Source: CAD feature listing. Evaluate the final solid. Frame: model axes, mm. Give positions to 0.01 mm unless a question says otherwise; leave off trailing zeros. Order: outer loops, then holes, each group sorted by start corner. A loop starts at its lowest first (then second) coordinate and runs counter-clockwise, first axis right, second up.
Autodesk Fusion 360 part; units mm, degrees
sketch "Sketch1" plane through (0, 0, 0) normal (0, 1, 0) x (1, 0, 0)
  line L0 (0, 0) -> (120, 0)
  line L1 (120, 0) -> (120, -30)
  line L2 (120, -30) -> (0, -30)
  line L3 (0, -30) -> (0, 0)
  dimension "d3" = 120
  dimension "d4" = 30
extrude "Extrude1" add sketch "Sketch1" along normal blind 3
sketch "Sketch3" plane through (0, 0, 0) normal (0, 1, 0) x (1, 0, 0)
  line L0 (120, -30) -> (0, -30)
  line L1 (0, -30) -> (0, 0)
  line L2 (0, 0) -> (120, 0)
  line L3 (120, 0) -> (120, -30)
  line L4 (0, -26.25) -> (-3, -26.25)
  line L5 (-3, -26.25) -> (-3, -18.75)
  line L6 (-3, -18.75) -> (0, -18.75)
  line L7 (0, -18.75) -> (0, -26.25)
  line L8 (0, -11.25) -> (-3, -11.25)
  line L9 (-3, -11.25) -> (-3, -3.75)
  line L10 (-3, -3.75) -> (0, -3.75)
  line L11 (0, -3.75) -> (0, -11.25)
  line L12 (3.75, 0) -> (11.25, 0)
  line L13 (11.25, 0) -> (11.25, 3)
  line L14 (11.25, 3) -> (3.75, 3)
  line L15 (3.75, 3) -> (3.75, 0)
  line L16 (18.75, 0) -> (26.25, 0)
  line L17 (26.25, 0) -> (26.25, 3)
  line L18 (26.25, 3) -> (18.75, 3)
  line L19 (18.75, 3) -> (18.75, 0)
  line L20 (116.25, 0) -> (108.75, 0)
  line L21 (108.75, 0) -> (108.75, 3)
  line L22 (108.75, 3) -> (116.25, 3)
  line L23 (116.25, 3) -> (116.25, 0)
  line L24 (101.25, 0) -> (93.75, 0)
  line L25 (93.75, 0) -> (93.75, 3)
  line L26 (93.75, 3) -> (101.25, 3)
  line L27 (101.25, 3) -> (101.25, 0)
  line L28 (120, -4.6509) -> (123, -4.6509)
  line L29 (123, -4.6509) -> (123, -12.1509)
  line L30 (123, -12.1509) -> (120, -12.1509)
  line L31 (120, -12.1509) -> (120, -4.6509)
  line L32 (120, -19.6509) -> (123, -19.6509)
  line L33 (123, -19.6509) -> (123, -27.1509)
  line L34 (123, -27.1509) -> (120, -27.1509)
  line L35 (120, -27.1509) -> (120, -19.6509)
  line L36 (116.25, -30) -> (108.75, -30)
  line L37 (108.75, -30) -> (108.75, -33)
  line L38 (108.75, -33) -> (116.25, -33)
  line L39 (116.25, -33) -> (116.25, -30)
  line L40 (101.25, -30) -> (93.75, -30)
  line L41 (93.75, -30) -> (93.75, -33)
  line L42 (93.75, -33) -> (101.25, -33)
  line L43 (101.25, -33) -> (101.25, -30)
  line L44 (26.25, -30) -> (18.75, -30)
  line L45 (18.75, -30) -> (18.75, -33)
  line L46 (18.75, -33) -> (26.25, -33)
  line L47 (26.25, -33) -> (26.25, -30)
  line L48 (11.25, -30) -> (3.75, -30)
  line L49 (3.75, -30) -> (3.75, -33)
  line L50 (3.75, -33) -> (11.25, -33)
  line L51 (11.25, -33) -> (11.25, -30)
  line L52 (3.75, 3) -> (0, 3) construction
  line L53 (11.25, 3) -> (18.75, 3) construction
  line L54 (101.25, 3) -> (108.75, 3) construction
  line L55 (116.25, 3) -> (120, 3) construction
  line L56 (120, 0) -> (120, -4.6509) construction
  line L57 (123, -12.1509) -> (123, -19.6509) construction
  line L58 (108.75, -33) -> (101.25, -33) construction
  line L59 (120, -30) -> (116.25, -30) construction
  dimension "d10" = 3
  dimension "d11" = 7.5
  dimension "d13" = 3
  dimension "d14" = 3.75
  dimension "d15" = 3.75
  dimension "d16" = 7.5
  dimension "d17" = 7.5
  dimension "d18" = 3.75
  dimension "d19" = 3.75
  dimension "d20" = 7.5
  dimension "d21" = 7.5
  dimension "d22" = 3.75
  dimension "d23" = 7.5
  dimension "d24" = 7.5
  dimension "d25" = 3.75
extrude "Extrude2" add sketch "Sketch3" along normal blind 3 contours L0 L36 L37 L38 L39 | L3 L32 L33 L34 L35 | L0 L40 L41 L42 L43 | L3 L28 L29 L30 L31 | L0 L44 L45 L46 L47 | L2 L20 L21 L22 L23 | L0 L48 L49 L50 L51 | L2 L24 L25 L26 L27 | L1 L4 L5 L6 L7 | L2 L16 L17 L18 L19 | L1 L8 L9 L10 L11 | L2 L12 L13 L14 L15
sketch "Sketch4" plane through (0, 0, 0) normal (0, 1, 0) x (1, 0, 0)
  line L0 (120, -30) -> (116.25, -30)
  line L1 (116.25, -30) -> (116.25, -33)
  line L2 (116.25, -33) -> (108.75, -33)
  line L3 (108.75, -33) -> (108.75, -30)
  line L4 (108.75, -30) -> (101.25, -30)
  line L5 (101.25, -30) -> (101.25, -33)
  line L6 (101.25, -33) -> (93.75, -33)
  line L7 (93.75, -33) -> (93.75, -30)
  line L8 (93.75, -30) -> (26.25, -30)
  line L9 (26.25, -30) -> (26.25, -33)
  line L10 (26.25, -33) -> (18.75, -33)
  line L11 (18.75, -33) -> (18.75, -30)
  line L12 (18.75, -30) -> (11.25, -30)
  line L13 (11.25, -30) -> (11.25, -33)
  line L14 (11.25, -33) -> (3.75, -33)
  line L15 (3.75, -33) -> (3.75, -30)
  line L16 (3.75, -30) -> (0, -30)
  line L17 (0, -30) -> (0, -26.25)
  line L18 (0, -26.25) -> (-3, -26.25)
  line L19 (-3, -26.25) -> (-3, -18.75)
  line L20 (-3, -18.75) -> (0, -18.75)
  line L21 (0, -18.75) -> (0, -11.25)
  line L22 (0, -11.25) -> (-3, -11.25)
  line L23 (-3, -11.25) -> (-3, -3.75)
  line L24 (-3, -3.75) -> (0, -3.75)
  line L25 (0, -3.75) -> (0, 0)
  line L26 (0, 0) -> (3.75, 0)
  line L27 (3.75, 0) -> (3.75, 3)
  line L28 (3.75, 3) -> (11.25, 3)
  line L29 (11.25, 3) -> (11.25, 0)
  line L30 (11.25, 0) -> (18.75, 0)
  line L31 (18.75, 0) -> (18.75, 3)
  line L32 (18.75, 3) -> (26.25, 3)
  line L33 (26.25, 3) -> (26.25, 0)
  line L34 (26.25, 0) -> (93.75, 0)
  line L35 (93.75, 0) -> (93.75, 3)
  line L36 (93.75, 3) -> (101.25, 3)
  line L37 (101.25, 3) -> (101.25, 0)
  line L38 (101.25, 0) -> (108.75, 0)
  line L39 (108.75, 0) -> (108.75, 3)
  line L40 (108.75, 3) -> (116.25, 3)
  line L41 (116.25, 3) -> (116.25, 0)
  line L42 (116.25, 0) -> (120, 0)
  line L43 (120, 0) -> (120, -4.6509)
  line L44 (120, -4.6509) -> (123, -4.6509)
  line L45 (123, -4.6509) -> (123, -12.1509)
  line L46 (123, -12.1509) -> (120, -12.1509)
  line L47 (120, -12.1509) -> (120, -19.6509)
  line L48 (120, -19.6509) -> (123, -19.6509)
  line L49 (123, -19.6509) -> (123, -27.1509)
  line L50 (123, -27.1509) -> (120, -27.1509)
  line L51 (120, -27.1509) -> (120, -30)
  line L52 (116.25, 0) -> (116.25, -30) construction
  line L53 (120, -27.1509) -> (0, -26.25) construction
  line L54 (0, -18.75) -> (120, -19.6509) construction
  line L55 (120, -12.1509) -> (0, -11.25) construction
  line L56 (0, -3.75) -> (120, -4.6509) construction
  line L57 (108.75, 0) -> (108.75, -30) construction
  line L58 (101.25, -30) -> (101.25, 0) construction
  line L59 (93.75, 0) -> (93.75, -30) construction
  line L60 (26.25, -30) -> (26.25, 0) construction
  line L61 (18.75, 0) -> (18.75, -30) construction
  line L62 (11.25, -30) -> (11.25, 0) construction
  line L63 (3.75, 0) -> (3.75, -30) construction
  line L64 (116.25, -4.6227) -> (113.25, -4.6227)
  line L65 (113.25, -4.6227) -> (113.25, -12.1002)
  line L66 (113.25, -12.1002) -> (116.25, -12.1002)
  line L67 (116.25, -12.1002) -> (116.25, -4.6227)
  line L68 (108.75, -4.5664) -> (116.25, -4.5664)
  line L69 (116.25, -4.5664) -> (116.25, -7.5664)
  line L70 (116.25, -7.5664) -> (108.75, -7.5664)
  line L71 (108.75, -7.5664) -> (108.75, -4.5664)
  line L72 (101.25, -4.5101) -> (93.75, -4.5101)
  line L73 (93.75, -4.5101) -> (93.75, -7.5101)
  line L74 (93.75, -7.5101) -> (101.25, -7.5101)
  line L75 (101.25, -7.5101) -> (101.25, -4.5101)
  line L76 (116.25, -19.6227) -> (113.25, -19.6227)
  line L77 (113.25, -19.6227) -> (113.25, -27.1002)
  line L78 (113.25, -27.1002) -> (116.25, -27.1002)
  line L79 (116.25, -27.1002) -> (116.25, -19.6227)
  line L80 (108.75, -27.0664) -> (116.25, -27.0664)
  line L81 (116.25, -27.0664) -> (116.25, -24.0664)
  line L82 (116.25, -24.0664) -> (108.75, -24.0664)
  line L83 (108.75, -24.0664) -> (108.75, -27.0664)
  line L84 (101.25, -27.0101) -> (93.75, -27.0101)
  line L85 (93.75, -27.0101) -> (93.75, -24.0101)
  line L86 (93.75, -24.0101) -> (101.25, -24.0101)
  line L87 (101.25, -24.0101) -> (101.25, -27.0101)
  line L88 (26.25, -26.4471) -> (18.75, -26.4471)
  line L89 (18.75, -26.4471) -> (18.75, -23.4471)
  line L90 (18.75, -23.4471) -> (26.25, -23.4471)
  line L91 (26.25, -23.4471) -> (26.25, -26.4471)
  line L92 (11.25, -26.3345) -> (3.75, -26.3345)
  line L93 (3.75, -26.3345) -> (3.75, -23.3345)
  line L94 (3.75, -23.3345) -> (11.25, -23.3345)
  line L95 (11.25, -23.3345) -> (11.25, -26.3345)
  line L96 (3.75, -18.7782) -> (6.75, -18.7782)
  line L97 (6.75, -18.7782) -> (6.75, -26.3345)
  line L98 (6.75, -26.3345) -> (3.75, -26.3345)
  line L99 (3.75, -26.3345) -> (3.75, -18.7782)
  line L100 (3.75, -11.2782) -> (6.75, -11.2782)
  line L101 (6.75, -11.2782) -> (6.75, -3.8007)
  line L102 (6.75, -3.8007) -> (3.75, -3.8007)
  line L103 (3.75, -3.8007) -> (3.75, -11.2782)
  line L104 (3.75, -3.8007) -> (11.25, -3.8007)
  line L105 (11.25, -3.8007) -> (11.25, -6.8007)
  line L106 (11.25, -6.8007) -> (3.75, -6.8007)
  line L107 (3.75, -6.8007) -> (3.75, -3.8007)
  line L108 (18.75, -3.8908) -> (26.25, -3.8908)
  line L109 (26.25, -3.8908) -> (26.25, -6.8908)
  line L110 (26.25, -6.8908) -> (18.75, -6.8908)
  line L111 (18.75, -6.8908) -> (18.75, -3.8908)
  dimension "d28" = 3
  dimension "d29" = 3
  dimension "d30" = 3
  dimension "d31" = 3
  dimension "d32" = 3
  dimension "d33" = 3
extrude "Extrude3" cut sketch "Sketch4" along normal up to surface (3 mm away) contours L64 L65 L67 L69 L70 | L64 L65 L68 L69 L70 L71 | L65 L66 L67 L70 | L72 L73 L74 L75 | L76 L77 L79 L82 | L77 L79 L80 L81 L82 | L77 L80 L82 L83 | L84 L85 L86 L87 | L88 L89 L90 L91 | L92 L94 L95 L97 | L92 L93 L94 L97 L98 L99 | L94 L96 L97 L99 | L100 L101 L103 L106 | L101 L102 L103 L104 L106 L107 | L101 L104 L105 L106 | L108 L109 L110 L111
equation "main_length = 120 mm"
equation "main_width = 30 mm"
equation "d3 = main_length"
equation "d4 = main_width"
equation "material_thickness = 3 mm"
equation "d6 = material_thickness"
equation "fit_length = 7.5 mm"
equation "fit_spacing = 7.5 mm"
equation "d10 = material_thickness"
equation "d11 = fit_length"
equation "d13 = material_thickness"
equation "d14 = fit_spacing / 2"
equation "d15 = fit_spacing / 2"
equation "d16 = fit_spacing"
equation "d17 = fit_spacing"
equation "d19 = fit_spacing / 2"
equation "d20 = fit_spacing"
equation "d21 = fit_spacing"
equation "d22 = fit_spacing / 2"
equation "d23 = fit_spacing"
equation "d24 = fit_spacing"
equation "d25 = fit_spacing / 2"
equation "d28 = material_thickness"
equation "d29 = material_thickness"
equation "d30 = material_thickness"
equation "d31 = material_thickness"
equation "d32 = material_thickness"
equation "d33 = material_thickness"
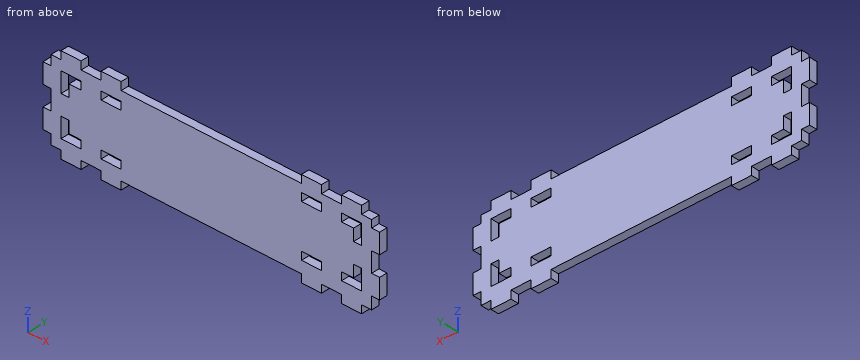
1) Section query B-B, the plane z = 21. Return the cut outline in (x, y).
Report:
outline: (-3, 0) - (3.75, 0) - (3.75, 3) - (-3, 3) - close; (6.75, 0) - (113.25, 0) - (113.25, 3) - (6.75, 3) - close; (116.25, 0) - (123, 0) - (123, 3) - (116.25, 3) - close
2) Section query D-D, the plane y = 1.6. Count the separate pieces of the cut face and the enclosed holes in it, and give its area (3 significant figures).
Report:
separate pieces: 1
enclosed holes: 8
area: 3,640 mm2
3) Material intervals for L1, parallel to X at y = 0.55, z = 8.5; L2, parallel to X at y = 2.6, z = 6; L3, parallel to Z at x = 20, y = 0.85, sorted ascending.
Report:
L1: x = -3 to 3.75, 6.75 to 113.25, 116.25 to 123
L2: x = -3 to 3.75, 11.25 to 18.75, 26.25 to 93.75, 101.25 to 108.75, 116.25 to 123
L3: z = -3 to 3.89, 6.89 to 23.45, 26.45 to 33
4) Section query A-A, the plane x = 111. Return the cut outline in (y, z), and give its area (3 significant figures).
Report:
outline: (0, -3) - (3, -3) - (3, 4.57) - (0, 4.57) - close; (0, 7.57) - (3, 7.57) - (3, 24.07) - (0, 24.07) - close; (0, 27.07) - (3, 27.07) - (3, 33) - (0, 33) - close
area: 90.0 mm2
5) Section query C-C, the plane x = 43.5. Return the cut outline in (y, z), and give its area (3 significant figures).
Report:
outline: (0, 0) - (3, 0) - (3, 30) - (0, 30) - close
area: 90.0 mm2
6) Pin query (flat end, axial travel): pin 1 (1 mm diameter, centred on y = 0.5, z = 3, fed in from +X); pin 2 (1.5 mm diameter, centred on y = 1.5, z = -2, fed in from -X); pin 3 (1.5 mm diameter, centred on y = 1.5, z = 32, fed in from +X). Return the tip coordinate at first contact, or that it passes through.
Report:
pin 1: stops at x = 120
pin 2: stops at x = 3.75
pin 3: stops at x = 116.25
